Design review of the part shown in the three views and the two pictorial views. Dimensions are in mm from the part's minimum x, y and z. Round coordinates to 2 decimals unless told otherwise and drop trailing zeros. Loops run counter-clockwise (first coordinate to the right, second up) from the corner with the lowest first, then second, coordinate; pieces in that order, holes last. Notation, with made-up numbers: (67, 85.25) -> (123, 85.25) arc R23 ccw to (123, 114.25) -> close; hole circle Ø10 at (65, 60). An arc over 180 degrees is marked (long way). One line per question, with ' | ' between items. Start each with the question number.
1. Draft analysis for pull direction X (two halves, no side actions). For the marked faces 1, 2 and 3, state which applies: pulls with the +X half, pulls with the -X half, needs draft (parallel to the pull), parting line crosses it, or undercut.
2. Wall thickness on line 1 along Z through (x, y) = (7, 0.4); line 2 along X through (y, z) = (1.6, 12.75); line 3 along Z through (x, y) = (19, 1.4) (1 decimal): over which ranges is each line inside the solid? List them lowest first.
3. Consider section A-A (x = 20.5). Write out the cut boundary in (y, z).
4. Consider section D-D (y = 0.85). Write out the cut boundary in (x, z).
5. Consider section C-C (z = 5). Write out the cut boundary in (x, y), and give its area (3 significant figures).
6. Consider section B-B (z = 12.75). Write out the cut boundary in (x, y).
7. For pin 1 Ø5 at (x, z) = (24, 24.5) entering from -Y, flat-tipped, find the tip position at first contact; note if it passes through.
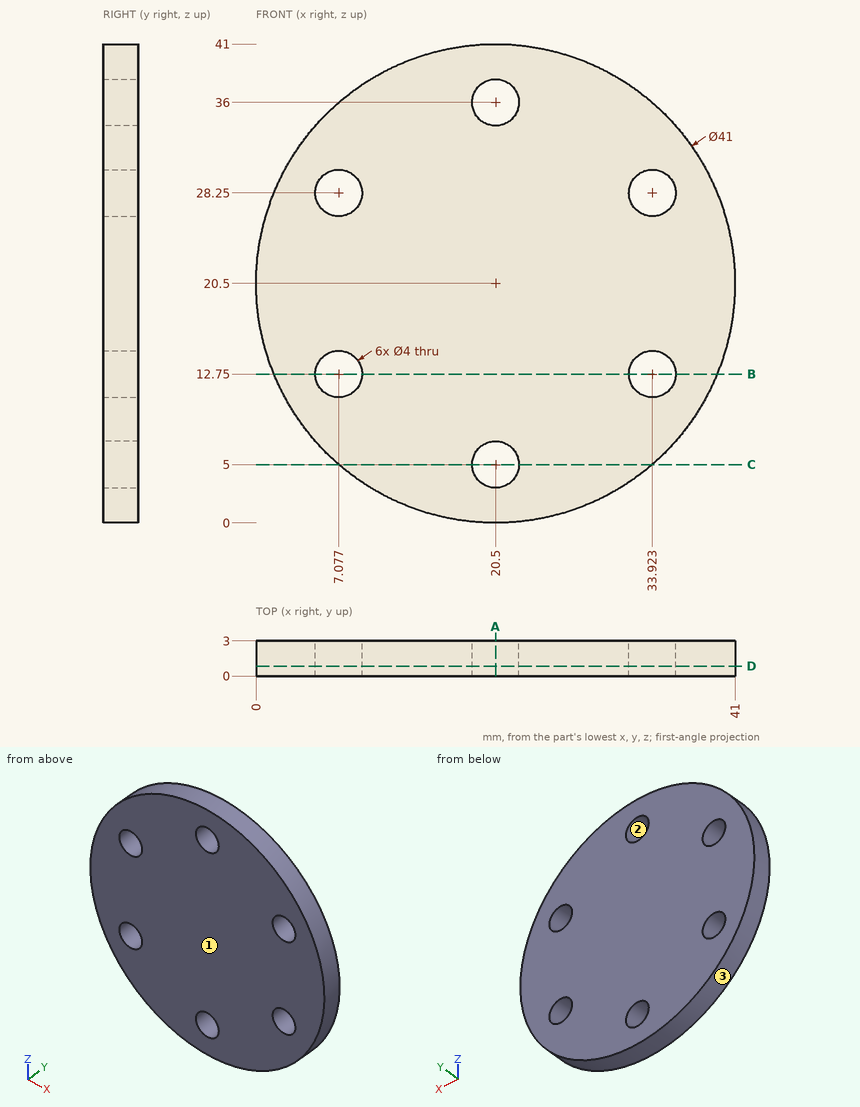
Answer block:
1) face 1: needs draft | face 2: undercut | face 3: parting line crosses it
2) line 1: z = 5.07 to 10.75, 14.75 to 26.25, 30.25 to 35.93 | line 2: x = 1.52 to 5.08, 9.08 to 31.92, 35.92 to 39.48 | line 3: z = 0.1 to 3.7, 6.3 to 34.7, 37.3 to 40.9
3) outline: (0, 0) -> (3, 0) -> (3, 3) -> (0, 3) -> close; (0, 7) -> (3, 7) -> (3, 34) -> (0, 34) -> close; (0, 38) -> (3, 38) -> (3, 41) -> (0, 41) -> close
4) outline: circle Ø41 at (20.5, 20.5); hole circle Ø4 at (7.08, 12.75); hole circle Ø4 at (7.08, 28.25); hole circle Ø4 at (20.5, 5); hole circle Ø4 at (20.5, 36); hole circle Ø4 at (33.92, 12.75); hole circle Ø4 at (33.92, 28.25)
5) outline: (7.08, 0) -> (18.5, 0) -> (18.5, 3) -> (7.08, 3) -> close; (22.5, 0) -> (33.92, 0) -> (33.92, 3) -> (22.5, 3) -> close | area: 68.5 mm2
6) outline: (1.52, 0) -> (5.08, 0) -> (5.08, 3) -> (1.52, 3) -> close; (9.08, 0) -> (31.92, 0) -> (31.92, 3) -> (9.08, 3) -> close; (35.92, 0) -> (39.48, 0) -> (39.48, 3) -> (35.92, 3) -> close
7) pin 1: stops at y = 0
